from build123d import *

# Parameters (mm, degrees)
PAD006_DEPTH            = 12
THICKNESS_T             = -1.6
POCKET005_DEPTH         = 0.4
BODY005_PLACEMENT_ANGLE = 30


with BuildPart() as part:
    # Sketch011 → Pad006 (new body)
    with BuildSketch(Plane.XY):
        with BuildLine():
            Line((-39.5, 29), (-39.5, -29))
            ThreePointArc((-39.5, -29), (-38.62132, -31.12132), (-36.5, -32))
            Line((-36.5, -32), (36.5, -32))
            ThreePointArc((36.5, -32), (38.62132, -31.12132), (39.5, -29))
            Line((39.5, -29), (39.5, 29))
            ThreePointArc((39.5, 29), (38.62132, 31.12132), (36.5, 32))
            Line((36.5, 32), (-36.5, 32))
            ThreePointArc((-36.5, 32), (-38.62132, 31.12132), (-39.5, 29))
        make_face()
    extrude(amount=PAD006_DEPTH)

    # Thickness
    thickness_openings = [part.faces().sort_by_distance(p)[0] for p in [
        (0, 0, 0),
    ]]
    offset(amount=THICKNESS_T, openings=thickness_openings)

    # Sketch012 (on Face9 of Thickness) → Pocket005 (cut)
    with BuildSketch(Plane(origin=(-25, 7, 12), x_dir=(0, 1, 0), z_dir=(0, 0, 1))):
        with BuildLine():
            Line((-31.53, -9.43), (-31.53, 5.57))
            Line((-31.53, 5.57), (-28.545807, 5.57))
            Line((-28.545807, 5.57), (-24.999522, -5.053183))
            add(Edge.make_bspline(
                [(-24.999522, -5.053183), (-24.50897, -6.537104), (-24.284133, -7.273614)],
                knots=[0, 0, 0, 1, 1, 1], degree=2))
            add(Edge.make_bspline(
                [(-24.284133, -7.273614), (-24.028637, -6.454664), (-23.486986, -4.868545)],
                knots=[0, 0, 0, 1, 1, 1], degree=2))
            Line((-23.486986, -4.868545), (-19.899822, 5.57))
            Line((-19.899822, 5.57), (-17.232444, 5.57))
            Line((-17.232444, 5.57), (-17.232444, -9.43))
            Line((-17.232444, -9.43), (-19.143554, -9.43))
            Line((-19.143554, -9.43), (-19.143554, 3.127458))
            Line((-19.143554, 3.127458), (-23.497206, -9.43))
            Line((-23.497206, -9.43), (-25.285678, -9.43))
            Line((-25.285678, -9.43), (-29.61889, 3.342075))
            Line((-29.61889, 3.342075), (-29.61889, -9.43))
            Line((-29.61889, -9.43), (-31.53, -9.43))
        make_face()
        with BuildLine():
            Line((-7.843817, -9.43), (-9.683388, -9.43))
            Line((-9.683388, -9.43), (-9.683388, 2.326223))
            add(Edge.make_bspline(
                [(-9.683388, 2.326223), (-10.347678, 1.695999), (-11.426212, 1.065094)],
                knots=[0, 0, 0, 1, 1, 1], degree=2))
            add(Edge.make_bspline(
                [(-11.426212, 1.065094), (-12.504064, 0.434871), (-13.362531, 0.119419)],
                knots=[0, 0, 0, 1, 1, 1], degree=2))
            Line((-13.362531, 0.119419), (-13.362531, 1.907209))
            add(Edge.make_bspline(
                [(-13.362531, 1.907209), (-11.819335, 2.630774), (-10.664493, 3.659571)],
                knots=[0, 0, 0, 1, 1, 1], degree=2))
            add(Edge.make_bspline(
                [(-10.664493, 3.659571), (-9.509651, 4.68905), (-9.029319, 5.657209)],
                knots=[0, 0, 0, 1, 1, 1], degree=2))
            Line((-9.029319, 5.657209), (-7.843817, 5.657209))
            Line((-7.843817, 5.657209), (-7.843817, -9.43))
        make_face()
        with BuildLine():
            Line((6.537542, -7.696715), (6.537542, -9.43))
            Line((6.537542, -9.43), (-3.365483, -9.43))
            add(Edge.make_bspline(
                [(-3.365483, -9.43), (-3.385923, -8.767754), (-3.150867, -8.155927)],
                knots=[0, 0, 0, 1, 1, 1], degree=2))
            add(Edge.make_bspline(
                [(-3.150867, -8.155927), (-2.772732, -7.146888), (-1.940156, -6.168508)],
                knots=[0, 0, 0, 1, 1, 1], degree=2))
            add(Edge.make_bspline(
                [(-1.940156, -6.168508), (-1.106899, -5.189448), (0.466957, -3.905154)],
                knots=[0, 0, 0, 1, 1, 1], degree=2))
            add(Edge.make_bspline(
                [(0.466957, -3.905154), (2.909499, -1.891165), (3.767965, -0.71452)],
                knots=[0, 0, 0, 1, 1, 1], degree=2))
            add(Edge.make_bspline(
                [(3.767965, -0.71452), (4.626432, 0.462124), (4.626432, 1.509998)],
                knots=[0, 0, 0, 1, 1, 1], degree=2))
            add(Edge.make_bspline(
                [(4.626432, 1.509998), (4.626432, 2.609653), (3.844273, 3.364559)],
                knots=[0, 0, 0, 1, 1, 1], degree=2))
            add(Edge.make_bspline(
                [(3.844273, 3.364559), (3.062796, 4.120145), (1.805756, 4.120145)],
                knots=[0, 0, 0, 1, 1, 1], degree=2))
            add(Edge.make_bspline(
                [(1.805756, 4.120145), (0.477177, 4.120145), (-0.319971, 3.312778)],
                knots=[0, 0, 0, 1, 1, 1], degree=2))
            add(Edge.make_bspline(
                [(-0.319971, 3.312778), (-1.117118, 2.506092), (-1.127338, 1.078721)],
                knots=[0, 0, 0, 1, 1, 1], degree=2))
            Line((-1.127338, 1.078721), (-3.018009, 1.274942))
            add(Edge.make_bspline(
                [(-3.018009, 1.274942), (-2.823832, 3.414295), (-1.556571, 4.535752)],
                knots=[0, 0, 0, 1, 1, 1], degree=2))
            add(Edge.make_bspline(
                [(-1.556571, 4.535752), (-0.289311, 5.657209), (1.846635, 5.657209)],
                knots=[0, 0, 0, 1, 1, 1], degree=2))
            add(Edge.make_bspline(
                [(1.846635, 5.657209), (4.003022, 5.657209), (5.260062, 4.454675)],
                knots=[0, 0, 0, 1, 1, 1], degree=2))
            add(Edge.make_bspline(
                [(5.260062, 4.454675), (6.517102, 3.25214), (6.517102, 1.474569)],
                knots=[0, 0, 0, 1, 1, 1], degree=2))
            add(Edge.make_bspline(
                [(6.517102, 1.474569), (6.517102, 0.570454), (6.149188, -0.303683)],
                knots=[0, 0, 0, 1, 1, 1], degree=2))
            add(Edge.make_bspline(
                [(6.149188, -0.303683), (5.781274, -1.177138), (4.927576, -2.143254)],
                knots=[0, 0, 0, 1, 1, 1], degree=2))
            add(Edge.make_bspline(
                [(4.927576, -2.143254), (4.07456, -3.108688), (2.091911, -4.794281)],
                knots=[0, 0, 0, 1, 1, 1], degree=2))
            add(Edge.make_bspline(
                [(2.091911, -4.794281), (0.436297, -6.193717), (-0.033815, -6.693127)],
                knots=[0, 0, 0, 1, 1, 1], degree=2))
            add(Edge.make_bspline(
                [(-0.033815, -6.693127), (-0.503928, -7.192536), (-0.810523, -7.696715)],
                knots=[0, 0, 0, 1, 1, 1], degree=2))
            Line((-0.810523, -7.696715), (6.537542, -7.696715))
        make_face()
        with BuildLine():
            add(Edge.make_bspline(
                [(8.512015, -2.02266), (8.512015, 0.643356), (9.058436, 2.26831)],
                knots=[0, 0, 0, 1, 1, 1], degree=2))
            add(Edge.make_bspline(
                [(9.058436, 2.26831), (9.605538, 3.893946), (10.68339, 4.775578)],
                knots=[0, 0, 0, 1, 1, 1], degree=2))
            add(Edge.make_bspline(
                [(10.68339, 4.775578), (11.761924, 5.657209), (13.397099, 5.657209)],
                knots=[0, 0, 0, 1, 1, 1], degree=2))
            add(Edge.make_bspline(
                [(13.397099, 5.657209), (14.60304, 5.657209), (15.512605, 5.170064)],
                knots=[0, 0, 0, 1, 1, 1], degree=2))
            add(Edge.make_bspline(
                [(15.512605, 5.170064), (16.422171, 4.682918), (17.014922, 3.765176)],
                knots=[0, 0, 0, 1, 1, 1], degree=2))
            add(Edge.make_bspline(
                [(17.014922, 3.765176), (17.607673, 2.848116), (17.944927, 1.530438)],
                knots=[0, 0, 0, 1, 1, 1], degree=2))
            add(Edge.make_bspline(
                [(17.944927, 1.530438), (18.282182, 0.21276), (18.282182, -2.02266)],
                knots=[0, 0, 0, 1, 1, 1], degree=2))
            add(Edge.make_bspline(
                [(18.282182, -2.02266), (18.282182, -4.667555), (17.740531, -6.29319)],
                knots=[0, 0, 0, 1, 1, 1], degree=2))
            add(Edge.make_bspline(
                [(17.740531, -6.29319), (17.198879, -7.918145), (16.120345, -8.805227)],
                knots=[0, 0, 0, 1, 1, 1], degree=2))
            add(Edge.make_bspline(
                [(16.120345, -8.805227), (15.042493, -9.691628), (13.397099, -9.691628)],
                knots=[0, 0, 0, 1, 1, 1], degree=2))
            add(Edge.make_bspline(
                [(13.397099, -9.691628), (11.230492, -9.691628), (9.993892, -8.133443)],
                knots=[0, 0, 0, 1, 1, 1], degree=2))
            add(Edge.make_bspline(
                [(9.993892, -8.133443), (8.512015, -6.25708), (8.512015, -2.02266)],
                knots=[0, 0, 0, 1, 1, 1], degree=2))
        make_face()
        with BuildLine():
            add(Edge.make_bspline(
                [(10.402685, -2.017209), (10.402685, -5.709978), (11.265921, -6.932271)],
                knots=[0, 0, 0, 1, 1, 1], degree=2))
            add(Edge.make_bspline(
                [(11.265921, -6.932271), (12.129838, -8.154564), (13.397099, -8.154564)],
                knots=[0, 0, 0, 1, 1, 1], degree=2))
            add(Edge.make_bspline(
                [(13.397099, -8.154564), (14.664359, -8.154564), (15.527595, -6.927502)],
                knots=[0, 0, 0, 1, 1, 1], degree=2))
            add(Edge.make_bspline(
                [(15.527595, -6.927502), (16.391512, -5.699758), (16.391512, -2.017209)],
                knots=[0, 0, 0, 1, 1, 1], degree=2))
            add(Edge.make_bspline(
                [(16.391512, -2.017209), (16.391512, 1.685779), (15.527595, 2.902622)],
                knots=[0, 0, 0, 1, 1, 1], degree=2))
            add(Edge.make_bspline(
                [(15.527595, 2.902622), (14.664359, 4.120145), (13.376659, 4.120145)],
                knots=[0, 0, 0, 1, 1, 1], degree=2))
            add(Edge.make_bspline(
                [(13.376659, 4.120145), (12.109399, 4.120145), (11.353131, 3.046381)],
                knots=[0, 0, 0, 1, 1, 1], degree=2))
            add(Edge.make_bspline(
                [(11.353131, 3.046381), (10.402685, 1.67556), (10.402685, -2.017209)],
                knots=[0, 0, 0, 1, 1, 1], degree=2))
        make_face(mode=Mode.SUBTRACT)
    extrude(amount=-POCKET005_DEPTH, mode=Mode.SUBTRACT)


with BuildPart() as part_1:
    # Body005 placement: moved
    add(part.part.moved(Location((34, -63.937892, 16.350669))).rotate(Axis((34, -63.937892, 16.350669), (1, 0, 0)), BODY005_PLACEMENT_ANGLE))


solid = part_1.part
Can you work these out from the model? Positions are in its coordinate system, mm. A direction names the side the tool comes from. Coordinates: 2 decimals unless noted, no trailing zeros. Write each loop counter-clockwise with the first axis right and the second up, starting at its lowest first coordinate (ties: lowest second). Pieces come first, ordered by that corner, then holes. Notation, with made-up numbers: (32.5, 77.25) - (62.5, 77.25) arc R15 cw to (62.5, 98.25) - close; hole circle Ø4 at (-37.75, 39). An arc over 180 degrees is marked (long way). Return JSON: item names as keys, results as strings. Group by question number.
Item 1: Please list where these lines run through material, in increasing order: probe 1 along X at (y, z) = (-57, 27); probe 2 along Y at (x, z) = (55.5, 39); probe 3 along Z at (x, y) = (12, -86).
Item 2: We'd pull the mould along Y, two halves only. Please class faces 4 (the face through (10.93, -52.24, 36.96)), 5 (the face through (8.722, -82.586, 19.213)), 6 (the face through (71.5, -40.54, 35.78)), 7 (the face through (-4.6, -39.9, 37)): pulls with the +Y half, pulls with the -Y half, needs draft (parallel to the pull), parting line crosses it, or undercut.
Item 3: Which directions (+Z, -Z, +X, -X, +Y, -Y) give clear straight access to the entire face, cutting with the end or side of a thin tool? Please do faces 1 (the face through (12.133, -87.525, 16.361)), 2 (the face through (12.063, -82.215, 19.427)), 3 (the face through (33.489, -94.609, 5.474)).
Item 4: I'm going to push flat-ended pins straight in: pin 1 Ø6 at (x, z) = (34, 10) entering from -Y; pin 2 Ø1 at (x, z) = (9.5, 34) entering from -Y; pin 3 Ø5 at (x, y) = (42, -45.5) entering from -Z. Where does each tip first touch, or does it pass through?
Item 5: If we section it at A-A (x = 43.5): Write out the boundary of the cut face in (y, z).
Return value:
{
 "1": {"probe 1": "x = -5.5 to -3.9, 71.9 to 73.5", "probe 2": "y = -48.71 to -45.51, -41.91 to -40.06", "probe 3": "z = 15.62 to 17.01, 17.19 to 17.47"},
 "2": {"face 4": "pulls with the -Y half", "face 5": "undercut", "face 6": "undercut", "face 7": "pulls with the +Y half"},
 "3": {"face 1": "+Z", "face 2": "-Y", "face 3": "-Z, +X, -X, -Y"},
 "4": {"pin 1": "stops at y = -97.65", "pin 2": "stops at y = -58.23", "pin 3": "stops at z = 37.56"},
 "5": {"outline": "(-97.65, 10.74) - (-91.65, 0.35) - (-90.27, 1.15) - (-95.47, 10.16) - (-42.81, 40.56) - (-37.61, 31.55) - (-36.23, 32.35) - (-42.23, 42.74) - close"}
}
